Work out the finished part from the listing and answer in its coordinate system (mm). A direction names the side the tool comes from. Give positions to 0.01 mm unless a question says otherwise; leave off trailing zeros. Order: outer loops, then holes, each group sorted by start corner. A loop starts at its lowest first (then second) coordinate and runs counter-clockwise, first axis right, second up. Notation, with made-up numbers: M 7.25,71 L 48.25,71 A29 cw 48.25,108 Z; hole C 78,-18 d6. An arc over 180 degrees is marked long. One line per item, written item: value.
from build123d import *

# Parameters (mm, degrees)
M14X1_5_TAPPED_HOLE1_D              = 12.5
M14X1_5_TAPPED_HOLE1_DEPTH          = 25.4
M14X1_5_TAPPED_HOLE1_TIP            = 3.755378869
F_1_16_0_0625_DIAMETER_HOLE1_D      = 1.5875
F_1_16_0_0625_DIAMETER_HOLE1_DEPTH  = 28.575
F_1_16_0_0625_DIAMETER_HOLE1_TIP    = 0.476933116
F_3_32_0_09375_DIAMETER_HOLE1_D     = 2.38125
F_3_32_0_09375_DIAMETER_HOLE1_DEPTH = 28.702
F_3_32_0_09375_DIAMETER_HOLE1_TIP   = 0.715399675
F_1_4_0_25_DIAMETER_HOLE1_D         = 6.35
CIRPATTERN1_COUNT                   = 6
F_1_32_0_03125_DIAMETER_HOLE1_D     = 0.79375
F_1_32_0_03125_DIAMETER_HOLE1_DEPTH = 28.575
F_1_32_0_03125_DIAMETER_HOLE1_TIP   = 0.238466558


with BuildPart() as part:
    # Sketch1 → Revolve1 (revolve)
    with BuildSketch(Plane.XY):
        Polygon((-12.7, 0), (-31.75, 0), (-31.75, 38.1), (-3.81, 38.1), (-3.81, 6.35), (-8.0645, 6.35), (-8.0645, 8.382), (-11.1125, 8.382), (-11.1125, 6.35), (-12.7, 6.35), align=None)
    revolve(axis=Axis((0, 0, 0), (0, 1, 0)))

    # M14x1.5 Tapped Hole1
    with Locations(Plane(origin=(0, 38.1, 0), x_dir=(1, 0, 0), z_dir=(0, 1, 0))):
        with Locations((0, 0)):
            Hole(M14X1_5_TAPPED_HOLE1_D / 2, depth=M14X1_5_TAPPED_HOLE1_DEPTH)
            with Locations((0, 0, -(M14X1_5_TAPPED_HOLE1_DEPTH + M14X1_5_TAPPED_HOLE1_TIP / 2))):  # 118° drill point
                Cone(0, M14X1_5_TAPPED_HOLE1_D / 2, M14X1_5_TAPPED_HOLE1_TIP, mode=Mode.SUBTRACT)

    # Sketch6 → 1/4 NPT Tapped Hole1 (revolve, cut)
    with BuildSketch(Plane(origin=(31.75, 19.05, 0), x_dir=(0, 0, -1), z_dir=(0, 1, 0))):
        Polygon((0, 0), (0, 20.360347279), (5.5626, 17.018), (5.5626, 9.906), (5.943685794, 9.906), (6.2402847, 0), align=None)
    revolve(axis=Axis((38.1, 19.05, 0), (-1, 0, 0)), mode=Mode.SUBTRACT)

    # Sketch8 → 1/4 NPT Tapped Hole2 (revolve, cut)
    with BuildSketch(Plane(origin=(-31.75, 19.05, 0), x_dir=(0, 0, 1), z_dir=(0, 1, 0))):
        Polygon((0, 0), (0, 20.360347279), (5.5626, 17.018), (5.5626, 9.906), (5.943685794, 9.906), (6.2402847, 0), align=None)
    revolve(axis=Axis((-38.1, 19.05, 0), (1, 0, 0)), mode=Mode.SUBTRACT)

    # 1/16 (0.0625) Diameter Hole1
    with Locations(Plane(origin=(31.75, 0, 0), x_dir=(0, 0, -1), z_dir=(1, 0, 0))):
        with Locations((0, 19.05)):
            Hole(F_1_16_0_0625_DIAMETER_HOLE1_D / 2, depth=F_1_16_0_0625_DIAMETER_HOLE1_DEPTH)
            with Locations((0, 0, -(F_1_16_0_0625_DIAMETER_HOLE1_DEPTH + F_1_16_0_0625_DIAMETER_HOLE1_TIP / 2))):  # 118° drill point
                Cone(0, F_1_16_0_0625_DIAMETER_HOLE1_D / 2, F_1_16_0_0625_DIAMETER_HOLE1_TIP, mode=Mode.SUBTRACT)

    # 3/32 (0.09375) Diameter Hole1
    with Locations(Plane.ZY.offset(31.75)):
        with Locations((0, 19.05)):
            Hole(F_3_32_0_09375_DIAMETER_HOLE1_D / 2, depth=F_3_32_0_09375_DIAMETER_HOLE1_DEPTH)
            with Locations((0, 0, -(F_3_32_0_09375_DIAMETER_HOLE1_DEPTH + F_3_32_0_09375_DIAMETER_HOLE1_TIP / 2))):  # 118° drill point
                Cone(0, F_3_32_0_09375_DIAMETER_HOLE1_D / 2, F_3_32_0_09375_DIAMETER_HOLE1_TIP, mode=Mode.SUBTRACT)

    # 1/4 (0.25) Diameter Hole1 (through all)
    with Locations(Plane(origin=(0, 38.1, 0), x_dir=(1, 0, 0), z_dir=(0, 1, 0))):
        with Locations((21.997045256, 12.7)):
            f_1_4_0_25_diameter_hole1 = Hole(F_1_4_0_25_DIAMETER_HOLE1_D / 2)

    # CirPattern1: 1/4 (0.25) Diameter Hole1 ×6 about axis
    cirpattern1_axis = Axis((0, 0, 0), (0, 1, 0))
    for i in range(1, CIRPATTERN1_COUNT):
        add(f_1_4_0_25_diameter_hole1.rotate(cirpattern1_axis, i * 360 / CIRPATTERN1_COUNT), mode=Mode.SUBTRACT)

    # Sketch18 → 1/4 NPT Tapped Hole3 (revolve, cut)
    with BuildSketch(Plane(origin=(15.875, 19.05, -27.49630657), x_dir=(-0.866025404, 0, -0.5), z_dir=(0, 1, 0))):
        Polygon((0, 0), (0, 20.360347279), (5.5626, 17.018), (5.5626, 9.906), (5.943685794, 9.906), (6.2402847, 0), align=None)
    revolve(axis=Axis((19.05, 19.05, -32.995567884), (-0.5, 0, 0.866025404)), mode=Mode.SUBTRACT)

    # 1/32 (0.03125) Diameter Hole1
    with Locations(Plane(origin=(15.875, 0, -27.49630657), x_dir=(0, -1, 0), z_dir=(0.5, 0, -0.866025404))):
        with Locations((-19.05, 0)):
            Hole(F_1_32_0_03125_DIAMETER_HOLE1_D / 2, depth=F_1_32_0_03125_DIAMETER_HOLE1_DEPTH)
            with Locations((0, 0, -(F_1_32_0_03125_DIAMETER_HOLE1_DEPTH + F_1_32_0_03125_DIAMETER_HOLE1_TIP / 2))):  # 118° drill point
                Cone(0, F_1_32_0_03125_DIAMETER_HOLE1_D / 2, F_1_32_0_03125_DIAMETER_HOLE1_TIP, mode=Mode.SUBTRACT)


solid = part.part
(1) Find the intervals of material crossed by probe 1 along Z at (x, y) = (0, 9) (3 decimals); probe 2 along Z at (x, y) = (0, 21) (3 decimals); probe 3 along Y at (x, z) = (-19.75, 0), in increasing order. Write a range as from..to.
Findings:
probe 1: z = -31.75..-28.575, -22.225..-3.81, 3.81..22.225, 28.575..31.75
probe 2: z = -31.75..-28.575, -22.225..-6.25, 6.25..22.225, 28.575..31.75
probe 3: y = 0..13.49, 24.61..38.1
(2) Section A-A, the plane z = 25.4 is taken. Give the vertices of the cut face in (x, y) (3 decimals), then the cut area to 3 significant figures.
Findings:
outline: M -19.05,0 L -3.175,0 L -3.175,38.1 L -19.05,38.1 Z; M 3.175,0 L 19.05,0 L 19.05,38.1 L 3.175,38.1 Z
area: 1,210 mm^2
(3) Which of the six approach directions +Z, -Z, +X, -X, +Y, -Y give full straight-line access (tool end or side, diameter ignored) to faces 3 (the cylindrical face through (-5.96, 25.22, -1.88)), 4 (the cylindrical face through (-10.6, 7.35, 3.34)), 5 (the flat face through (-21.844, 21.2, -5.3))?
Findings:
face 3: +Y
face 4: -Y
face 5: -X
(4) Section B-B, the plane x = 0 is taken. Give the number of separate pieces and of enclosed holes in the cut face, then the cut area to 3 significant figures.
Findings:
separate pieces: 4
enclosed holes: 0
area: 1,390 mm^2
(5) Determine the mould class of faces 1 (the flat face through (14, 0, 0)), 2 (the conical face through (-26.87, 18.78, -6.09)) for opening direction Z: pulls with the +Z half, pulls with the -Z half, needs draft (parallel to the pull), parting line crosses it, or undercut.
Findings:
face 1: needs draft
face 2: undercut
(6) Given P1, Ø2, axis at y = 19.05, z = 0, coming from the -X side; P2, Ø12, axis at x = -23.5, y = 25, coming from the -Z side; P3, Ø18, axis at x = 2.5, z = -0.5, coming from the -Y side, each flat-ended and moving along its own axis, determine where each tip first touches the part or whether it passes through.
Findings:
P1: stops at x = 6.17
P2: stops at z = -26.49
P3: stops at y = 6.35
